Verification items for the finished model (mm, model axes). A direction names the side the tool comes from. Give positions to 0.01 mm unless a question says otherwise; leave off trailing zeros. Loops run counter-clockwise (first coordinate to the right, second up) from the corner with the lowest first, then second, coordinate; pieces in that order, holes last. Notation, with made-up numbers: M 12.25,75.25 L 22.25,75.25 A12 ccw 22.25,92.25 Z; hole C 24,21.5 d4. An arc over 180 degrees is marked long. Put each result on its own line as item: value. Start each with the question number.
Autodesk Inventor part; units mm, degrees
ref_plane "YZ Plane" through (0, 0, 0) normal (1, 0, 0) x (0, 1, 0)
ref_plane "XZ Plane" through (0, 0, 0) normal (0, 1, 0) x (-1, 0, 0)
ref_plane "XY Plane" through (0, 0, 0) normal (0, 0, 1) x (1, 0, 0)
sketch "Sketch1" plane through (0, 0, 0) normal (0, 1, 0) x (-1, 0, 0)
  line L0 (32.1869, 7.2802) -> (22.6166, 4.1818)
  line L1 (-32.1869, 7.2802) -> (-22.6166, 4.1818)
  arc A0 (32.1869, 7.2802) -> (-32.1869, 7.2802) centre (0, 0) ccw
  arc A1 (22.6166, 4.1818) -> (-22.6166, 4.1818) centre (0, 0) ccw
  dimension "d7" = 23
  dimension "d8" = 33
extrude "Extrusion1" add sketch "Sketch1" along normal blind 10
sketch "Sketch2" plane through (0, 10, 0) normal (0, 1, 0) x (1, 0, 0)
  arc A0 (-32.1869, -7.2802) -> (32.1869, -7.2802) centre (0, 0) ccw
  line L0 (0, -35) -> (-16.5, -35)
  line L1 (-16.5, -35) -> (16.5, -35)
  line L2 (-16.5, -35) -> (-16.5, -28.5788)
  line L3 (16.5, -35) -> (16.5, -28.5788)
  dimension "d10" = 16.5
  dimension "d11" = 33
extrude "Extrusion2" add sketch "Sketch2" against normal blind 5
properties part number "g_jaws"
Q1. Go/stop test with flat-tipped pins: pin 1 (1.5 mm diameter, centred on x = -6.5, y = 7.5, fed in from -Z); pin 2 (1.5 mm diameter, centred on y = 7.5, z = 33, fed in from +X); pin 3 (5 mm diameter, centred on x = -0.5, z = 31, fed in from -Y); pin 4 (2.5 mm diameter, centred on y = 7.5, z = 31.5, fed in from -X). Record where each tip stops, or that it passes through.
Q2. Cross-section at B-B, the plane y = 6.25. Record the boundary of the cut face in (x, z).
Q3. Cross-section at A-A, the plane z = 10.5. Record the boundary of the cut face in (x, y).
Q4. Scan lines: L1, parallel to X at y = 7.75, z = 33; L2, parallel to X at y = 4, z = 12.5; L3, parallel to X at y = 6.5, z = 20.5. Record each from-to range of solid material in increasing order.
Q5. Cross-section at C-C, the plane z = 30. Record the boundary of the cut face in (x, y), then the cut area to 3 significant figures.
Q6. Cross-section at D-D, the plane x = -1. Record the boundary of the cut face in (y, z), then the cut area to 3 significant figures.
Q7. Release check for a two-part mould opening along X. For faces 5 (the face through (0, 5, 23)), 6 (the face through (0.623, 3.819, 32.994)), 7 (the face through (-27.469, 4.93, 5.753)) record: pulls with the +X half, pulls with the -X half, needs draft (parallel to the pull), parting line crosses it, or undercut.
Q8. Set-up check for faces 1 (the face through (16.5, 8, 32)), 2 (the face through (-16.5, 8, 32)), 3 (the face through (0, 0, 25)), 4 (the face through (-0.2, 5, 33.2)): record each of +Z, -Z, +X, -X, +Y, -Y from which the full face is reachable in a straight line by a thin tool's end or side.
Ans:
1. pin 1: stops at z = 21.83
1. pin 2: stops at x = 16.5
1. pin 3: stops at y = 0
1. pin 4: stops at x = -16.5
2. outline: M -32.19,7.28 L -22.62,4.18 A23 cw 22.62,4.18 L 32.19,7.28 A33 ccw 16.5,28.58 L 16.5,35 L -16.5,35 L -16.5,28.58 A33 ccw Z
3. outline: M -31.28,0 L -20.46,0 L -20.46,10 L -31.28,10 Z; M 20.46,0 L 31.28,0 L 31.28,10 L 20.46,10 Z
4. L1: x = -16.5 to 16.5
4. L2: x = -30.54 to -19.31, 19.31 to 30.54
4. L3: x = -25.86 to -10.43, 10.43 to 25.86
5. outline: M -16.5,5 L -13.75,5 L -13.75,0 L 13.75,0 L 13.75,5 L 16.5,5 L 16.5,10 L -16.5,10 Z
5. area: 302 mm^2
6. outline: M 0,22.98 L 10,22.98 L 10,35 L 5,35 L 5,32.98 L 0,32.98 Z
6. area: 110 mm^2
7. face 5: undercut
7. face 6: parting line crosses it
7. face 7: pulls with the -X half
8. face 1: +Z, +X, +Y, -Y
8. face 2: +Z, -X, +Y, -Y
8. face 3: +Z, -Z, +X, -X, -Y
8. face 4: +Z, -Y
